Here's how the part is built. I have some questions about the finished solid (model axes, mm). Give positions to 0.01 mm unless a question says otherwise; leave off trailing zeros. Order: outer loops, then holes, each group sorted by start corner. A loop starts at its lowest first (then second) coordinate and runs counter-clockwise, first axis right, second up. Notation, with made-up numbers: (73, 85.25) -> (77, 85.25) arc R20 ccw to (77, 99.25) -> close; hole circle Ø11 at (39, 37.5). An arc over 180 degrees is marked (long way). Write each question's results on one line, items separated by ' | '. Start each with the question number.
Q1. Imagine slicing it at B-B, the plane z = 0.95. Please give me the cut outline in (x, y) (3 decimals).
Q2. I need wall thicknesses on line 1 along X through (y, z) = (-5, 1.1) (3 decimals); line 2 along X through (y, z) = (-2, 0.9) (3 decimals); line 3 along Y through (x, z) = (4, 1.1). Which ranges of each line are inside material? Lowest first, please. Write a range as [from, to].
Q3. Imagine slicing it at A-A, the plane y = -5. Please give me the cut outline in (x, z) (3 decimals), then the cut area to 3 significant figures.
```python
from build123d import *

# Parameters (mm, degrees)
F0_W     = 15
F0_H     = 10
F1_DEPTH = 1.5748
F3_DEPTH = 25


with BuildPart() as f1:
    # F0 (on Top) → F1 (new body)
    with BuildSketch(Plane.XY):
        with Locations((0, -5)):
            Rectangle(F0_W, F0_H)
    extrude(amount=F1_DEPTH)

    # F2 (on face) → F3 (cut)
    with BuildSketch(Plane.XY.offset(1.5748)):
        with BuildLine():
            ThreePointArc((-4.435, -2.1), (-4.3178427125, -2.3828427125), (-4.035, -2.5))
            ThreePointArc((-4.035, -2.5), (-3.7521572875, -2.3828427125), (-3.635, -2.1))
            Line((-3.635, -2.1), (-3.635, -1.1))
            ThreePointArc((-3.635, -1.1), (-3.7521572875, -0.8171572875), (-4.035, -0.7))
            ThreePointArc((-4.035, -0.7), (-4.3178427125, -0.8171572875), (-4.435, -1.1))
            Line((-4.435, -1.1), (-4.435, -2.1))
        make_face()
        with BuildLine():
            ThreePointArc((-4.635, -5.8), (-4.5178427125, -6.0828427125), (-4.235, -6.2))
            ThreePointArc((-4.235, -6.2), (-3.9521572875, -6.0828427125), (-3.835, -5.8))
            Line((-3.835, -5.8), (-3.835, -4.8))
            ThreePointArc((-3.835, -4.8), (-3.9521572875, -4.5171572875), (-4.235, -4.4))
            ThreePointArc((-4.235, -4.4), (-4.5178427125, -4.5171572875), (-4.635, -4.8))
            Line((-4.635, -4.8), (-4.635, -5.8))
        make_face()
        with BuildLine():
            ThreePointArc((3.835, -5.8), (3.9521572875, -6.0828427125), (4.235, -6.2))
            ThreePointArc((4.235, -6.2), (4.5178427125, -6.0828427125), (4.635, -5.8))
            Line((4.635, -5.8), (4.635, -4.8))
            ThreePointArc((4.635, -4.8), (4.5178427125, -4.5171572875), (4.235, -4.4))
            ThreePointArc((4.235, -4.4), (3.9521572875, -4.5171572875), (3.835, -4.8))
            Line((3.835, -4.8), (3.835, -5.8))
        make_face()
        with BuildLine():
            ThreePointArc((4.035, -2.5), (4.3178427125, -2.3828427125), (4.435, -2.1))
            Line((4.435, -2.1), (4.435, -1.1))
            ThreePointArc((4.435, -1.1), (4.3178427125, -0.8171572875), (4.035, -0.7))
            ThreePointArc((4.035, -0.7), (3.7521572875, -0.8171572875), (3.635, -1.1))
            Line((3.635, -1.1), (3.635, -2.1))
            ThreePointArc((3.635, -2.1), (3.7521572875, -2.3828427125), (4.035, -2.5))
        make_face()
    extrude(amount=-F3_DEPTH, mode=Mode.SUBTRACT)


solid = f1.part
```
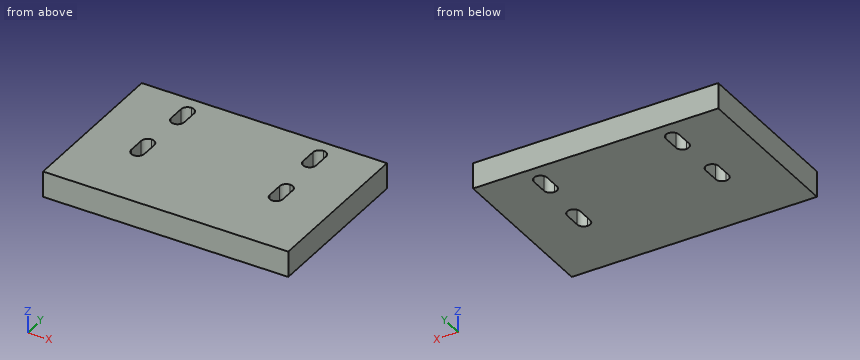
Geometry check:
1) outline: (-7.5, -10) -> (7.5, -10) -> (7.5, 0) -> (-7.5, 0) -> close; hole (-4.635, -5.8) arc R0.4 ccw to (-3.835, -5.8) -> (-3.835, -4.8) arc R0.4 ccw to (-4.635, -4.8) -> close; hole (-4.435, -2.1) arc R0.4 ccw to (-3.635, -2.1) -> (-3.635, -1.1) arc R0.4 ccw to (-4.435, -1.1) -> close; hole (3.635, -2.1) arc R0.4 ccw to (4.435, -2.1) -> (4.435, -1.1) arc R0.4 ccw to (3.635, -1.1) -> close; hole (3.835, -5.8) arc R0.4 ccw to (4.635, -5.8) -> (4.635, -4.8) arc R0.4 ccw to (3.835, -4.8) -> close
2) line 1: [-7.5, -4.635], [-3.835, 3.835], [4.635, 7.5] | line 2: [-7.5, -4.435], [-3.635, 3.635], [4.435, 7.5] | line 3: [-10, -6.12], [-4.48, -2.5], [-0.7, 0]
3) outline: (-7.5, 0) -> (-4.635, 0) -> (-4.635, 1.575) -> (-7.5, 1.575) -> close; (-3.835, 0) -> (3.835, 0) -> (3.835, 1.575) -> (-3.835, 1.575) -> close; (4.635, 0) -> (7.5, 0) -> (7.5, 1.575) -> (4.635, 1.575) -> close | area: 21.1 mm²
